Here's how the part is built. I have some questions about the finished solid (model axes, mm). A direction names the side the tool comes from. Round coordinates to 2 decimals unless told otherwise and drop trailing zeros. Write each loop counter-clockwise with the first axis right and the second up, starting at its lowest first coordinate (ties: lowest second). Pieces come first, ordered by that corner, then holes. Notation, with made-up numbers: (-35.5, 21.25) -> (22.5, 21.25) arc R25 cw to (22.5, 59.25) -> close; hole circle Ø7 at (61, 22.25). An arc over 180 degrees is marked (long way). Answer as CSV lines item,"result".
from build123d import *

# Parameters (mm, degrees)
F0_W     = 25
F0_H     = 25
F1_DEPTH = 150
F2_DEPTH = 150
F3_W     = 150
F3_H     = 50
F4_DEPTH = 810


with BuildPart() as f1:
    # F0 (on Front) → F1 (new body)
    with BuildSketch(Plane.XZ):
        Polygon((68.171213, 0), (68.171213, 50), (-31.828787, 50), (-31.828787, 25), (-6.828787, 25), (-6.828787, 0), align=None)
        with Locations((-44.328787, 37.5)):
            Rectangle(F0_W, F0_H)
        with Locations((-44.328787, 12.5)):
            Rectangle(F0_W, F0_H)
    extrude(amount=F1_DEPTH)

    # F0 (on Front) → F2 (join)
    with BuildSketch(Plane.XZ):
        Polygon((68.171213, 0), (68.171213, 50), (-31.828787, 50), (-31.828787, 25), (-6.828787, 25), (-6.828787, 0), align=None)
        with Locations((-44.328787, 37.5)):
            Rectangle(F0_W, F0_H)
        with Locations((-44.328787, 12.5)):
            Rectangle(F0_W, F0_H)
    extrude(amount=F2_DEPTH)

    # F3 (on face) → F4 (join)
    with BuildSketch(Plane.YZ.offset(68.171213)):
        with Locations((-75, 25)):
            Rectangle(F3_W, F3_H)
    extrude(amount=F4_DEPTH)


solid = f1.part
Item 1: Will this pin go through, and if not, where does the flat tip stop? pin 1 (2 mm diameter, centred on x = 86, y = -128.5, fed in from -Z).
Results found:
pin 1,"stops at z = 0"
Item 2: Suppose I cut it at A-A, the plane z = 16.5. List the corners of the cut face in (x, y) for me, then the cut area to 4 significant figures.
Results found:
outline,"(-56.83, -150) -> (-31.83, -150) -> (-31.83, 0) -> (-56.83, 0) -> close; (-6.83, -150) -> (878.17, -150) -> (878.17, 0) -> (-6.83, 0) -> close"
area,"136,500 mm²"
Item 3: If we mould it in two halves opening along X, with no side actions, what happens to faces 3 (the flat face through (-20, -74, 25)), 4 (the flat face through (878.171, -76, 25)), 5 (the flat face through (429, -76, 0))? For each: pulls with the +X half, pulls with the -X half, needs draft (parallel to the pull), parting line crosses it, or undercut.
Results found:
face 3,"undercut"
face 4,"pulls with the +X half"
face 5,"needs draft"
Item 4: I need wall thicknesses on L1, parallel to X at y = -30, z = 11; L2, parallel to Z at x = -19, y = -99. Which ranges of each line are inside material? Lowest first, please.
Results found:
L1,"x = -56.83 to -31.83, -6.83 to 878.17"
L2,"z = 25 to 50"
Item 5: For faces 1 (the flat face through (404, -150, 25)), 2 (the flat face through (-6.829, -74, 13)), which set-ups out of +Z, -Z, +X, -X, +Y, -Y let a thin tool reach every point of the face, with its end or its side?
Results found:
face 1,"+Z, -Z, +X, -X, -Y"
face 2,"-Z, +Y, -Y"
